from build123d import *

# Parameters (mm, degrees)
BOSS_EXTRUDE1_DEPTH = 100
BOSS_EXTRUDE2_DEPTH = 95
CUT_EXTRUDE1_DEPTH  = 5
BOSS_EXTRUDE5_DEPTH = 85
CUT_EXTRUDE4_DEPTH  = 5
BOSS_EXTRUDE6_DEPTH = 60
CUT_EXTRUDE5_DEPTH  = 40
SKETCH11_R          = 2.5
CUT_EXTRUDE6_DEPTH  = 15
SKETCH12_R          = 2.5
CUT_EXTRUDE7_DEPTH  = 15
CUT_EXTRUDE8_DEPTH  = 5
CUT_EXTRUDE9_DEPTH  = 30
CUT_EXTRUDE10_DEPTH = 5
CUT_EXTRUDE11_DEPTH = 30


with BuildPart() as part:
    # Sketch1 → Boss-Extrude1 (new body)
    with BuildSketch(Plane.XY):
        with BuildLine():
            Line((-70, 0), (-70, 30))
            Line((-70, 30), (-55, 45))
            Line((-55, 45), (-55, 55))
            Line((-55, 55), (-70, 70))
            Line((-70, 70), (-70, 100))
            ThreePointArc((-70, 100), (-35, 65), (0, 100))
            Line((0, 100), (0, 70))
            Line((0, 70), (-15, 55))
            Line((-15, 55), (-15, 45))
            Line((-15, 45), (0, 30))
            Line((0, 30), (0, 0))
            ThreePointArc((0, 0), (-35, 35), (-70, 0))
        make_face()
    extrude(amount=BOSS_EXTRUDE1_DEPTH)

    # Sketch2 → Boss-Extrude2 (add)
    with BuildSketch(Plane(origin=(0, 0, 0), x_dir=(-1, 0, 0), z_dir=(0, 0, -1))):
        with BuildLine():
            Line((0, 100), (10, 100))
            ThreePointArc((10, 100), (35, 75), (60, 100))
            Line((60, 100), (70, 100))
            ThreePointArc((70, 100), (35, 65), (0, 100))
        make_face()
        with BuildLine():
            Line((0, 0), (10, 0))
            ThreePointArc((10, 0), (35, 25), (60, 0))
            Line((60, 0), (70, 0))
            ThreePointArc((70, 0), (35, 35), (0, 0))
        make_face()
    extrude(amount=-BOSS_EXTRUDE2_DEPTH)

    # Sketch3 → Cut-Extrude1 (cut)
    with BuildSketch(Plane(origin=(0, 0, 0), x_dir=(-1, 0, 0), z_dir=(0, 0, -1))):
        with BuildLine():
            Line((0, 100), (10, 100))
            ThreePointArc((10, 100), (35, 75), (60, 100))
            Line((60, 100), (70, 100))
            ThreePointArc((70, 100), (35, 65), (0, 100))
        make_face()
        with BuildLine():
            Line((60, 0), (70, 0))
            ThreePointArc((70, 0), (35, 35), (0, 0))
            Line((0, 0), (10, 0))
            ThreePointArc((10, 0), (35, 25), (60, 0))
        make_face()
    extrude(amount=-CUT_EXTRUDE1_DEPTH, mode=Mode.SUBTRACT)

    # Sketch4 → Boss-Extrude5 (add)
    with BuildSketch(Plane(origin=(0, 0, 5), x_dir=(-1, 0, 0), z_dir=(0, 0, -1))):
        with BuildLine():
            Line((10, 100), (17.5, 100))
            ThreePointArc((17.5, 100), (35, 82.5), (52.5, 100))
            Line((52.5, 100), (60, 100))
            ThreePointArc((60, 100), (35, 75), (10, 100))
        make_face()
        with BuildLine():
            Line((10, 0), (17.5, 0))
            ThreePointArc((17.5, 0), (35, 17.5), (52.5, 0))
            Line((52.5, 0), (60, 0))
            ThreePointArc((60, 0), (35, 25), (10, 0))
        make_face()
    extrude(amount=-BOSS_EXTRUDE5_DEPTH)

    # Sketch7 → Cut-Extrude4 (cut)
    with BuildSketch(Plane(origin=(0, 0, 5), x_dir=(-1, 0, 0), z_dir=(0, 0, -1))):
        with BuildLine():
            ThreePointArc((52.5, 100), (35, 82.5), (17.5, 100))
            Line((17.5, 100), (10, 100))
            ThreePointArc((10, 100), (35, 75), (60, 100))
            Line((60, 100), (52.5, 100))
        make_face()
        with BuildLine():
            Line((10, 0), (17.5, 0))
            ThreePointArc((17.5, 0), (35, 17.5), (52.5, 0))
            Line((52.5, 0), (60, 0))
            ThreePointArc((60, 0), (35, 25), (10, 0))
        make_face()
    extrude(amount=-CUT_EXTRUDE4_DEPTH, mode=Mode.SUBTRACT)

    # Sketch9 → Boss-Extrude6 (add)
    with BuildSketch(Plane(origin=(0, 0, 0), x_dir=(-1, 0, 0), z_dir=(0, 0, -1))):
        Polygon((10, 40), (15, 45), (15, 55), (10, 60), align=None)
        Polygon((60, 60), (55, 55), (55, 45), (60, 40), align=None)
    extrude(amount=-BOSS_EXTRUDE6_DEPTH)

    # Sketch10 → Cut-Extrude5 (cut)
    with BuildSketch(Plane(origin=(0, 0, 0), x_dir=(-1, 0, 0), z_dir=(0, 0, -1))):
        Polygon((10, 40), (15, 45), (15, 55), (10, 60), align=None)
        Polygon((60, 40), (55, 45), (55, 55), (60, 60), align=None)
    extrude(amount=-CUT_EXTRUDE5_DEPTH, mode=Mode.SUBTRACT)

    # Sketch11 → Cut-Extrude6 (cut)
    with BuildSketch(Plane(origin=(-10, 0, 0), x_dir=(0, 0, -1), z_dir=(1, 0, 0))):
        with Locations((-50, 50)):
            Circle(SKETCH11_R)
    extrude(amount=-CUT_EXTRUDE6_DEPTH, mode=Mode.SUBTRACT)

    # Sketch12 → Cut-Extrude7 (cut)
    with BuildSketch(Plane.ZY.offset(60)):
        with Locations((50, 50)):
            Circle(SKETCH12_R)
    extrude(amount=-CUT_EXTRUDE7_DEPTH, mode=Mode.SUBTRACT)

    # Sketch13 → Cut-Extrude8 (cut)
    with BuildSketch(Plane(origin=(0, 0, 0), x_dir=(-1, 0, 0), z_dir=(0, 0, -1))):
        with BuildLine():
            Line((30, 60), (40, 60))
            ThreePointArc((40, 60), (50, 50), (40, 40))
            Line((40, 40), (30, 40))
            ThreePointArc((30, 40), (20, 50), (30, 60))
        make_face()
    extrude(amount=-CUT_EXTRUDE8_DEPTH, mode=Mode.SUBTRACT)

    # Sketch14 → Cut-Extrude9 (cut)
    with BuildSketch(Plane(origin=(0, 0, 5), x_dir=(-1, 0, 0), z_dir=(0, 0, -1))):
        with BuildLine():
            Line((30, 55), (40, 55))
            ThreePointArc((40, 55), (45, 50), (40, 45))
            Line((40, 45), (30, 45))
            ThreePointArc((30, 45), (25, 50), (30, 55))
        make_face()
    extrude(amount=-CUT_EXTRUDE9_DEPTH, mode=Mode.SUBTRACT)

    # Sketch15 → Cut-Extrude10 (cut)
    with BuildSketch(Plane.XY.offset(100)):
        with BuildLine():
            Line((-40, 60), (-30, 60))
            ThreePointArc((-30, 60), (-20, 50), (-30, 40))
            Line((-30, 40), (-40, 40))
            ThreePointArc((-40, 40), (-50, 50), (-40, 60))
        make_face()
    extrude(amount=-CUT_EXTRUDE10_DEPTH, mode=Mode.SUBTRACT)

    # Sketch16 → Cut-Extrude11 (cut)
    with BuildSketch(Plane.XY.offset(95)):
        with BuildLine():
            Line((-40, 55), (-30, 55))
            ThreePointArc((-30, 55), (-25, 50), (-30, 45))
            Line((-30, 45), (-40, 45))
            ThreePointArc((-40, 45), (-45, 50), (-40, 55))
        make_face()
    extrude(amount=-CUT_EXTRUDE11_DEPTH, mode=Mode.SUBTRACT)


solid = part.part
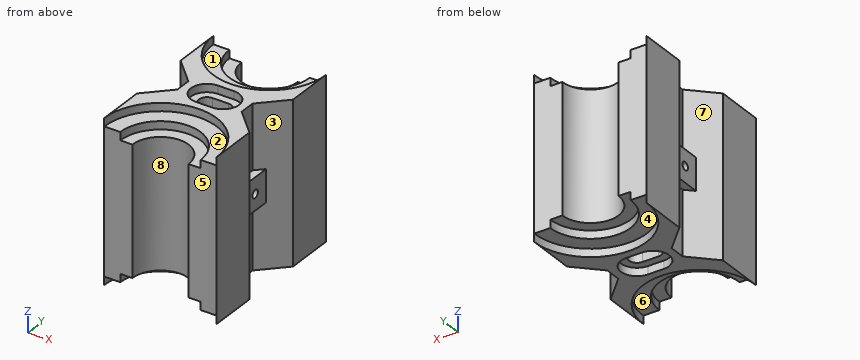
Check sheet for the modelled part. Datum: model origin and axes. Units: mm. Face numbers are marked on the shaded views. A direction names the side the tool comes from. Round coordinates to 2 decimals unless told otherwise and drop trailing zeros. Write each loop counter-clockwise with the first axis right and the second up, starting at its lowest first coordinate (ties: lowest second). Pieces come first, ordered by that corner, then holes. Notation, with made-up numbers: (69, 80.5) - (73, 80.5) arc R12 cw to (73, 97.5) - close; hole circle Ø9 at (86.5, 28.5). An arc over 180 degrees is marked (long way). Return JSON: item names as keys, results as strings.
Q1. Access from +Z, -Z, +X, -X, +Y, -Y to the whole of each face (thin tool, end or side, straight path). Record for the marked faces 1, 2, 3 and 4.
Returned:
{"face 1": "+Z, +Y", "face 2": "+Z, -Y", "face 3": "+X", "face 4": "-Z, +Y"}
Q2. Cross-section at B-B (x = -64.5). Record the boundary of the cut face in (y, z).
Returned:
{"outline": "(0, 5) - (18.83, 5) - (18.83, 0) - (35.5, 0) - (35.5, 100) - (18.83, 100) - (18.83, 95) - (0, 95) - close; (64.5, 0) - (81.17, 0) - (81.17, 5) - (100, 5) - (100, 95) - (81.17, 95) - (81.17, 100) - (64.5, 100) - close"}
Q3. Draft check along X on the marked faces 5, 6, 7 and 8. Enter one of: released by +X, released by -X, zero draft, split by the parting line, or undercut.
Returned:
{"face 5": "zero draft", "face 6": "undercut", "face 7": "released by -X", "face 8": "undercut"}
Q4. Scan lines: L1, parallel to Y at x = -53.5, z = 50; L2, parallel to Y at x = -34, z = 66; L3, parallel to Z at x = -45.5, y = 54. Record each from-to range of solid material in increasing order. Write a range as from..to.
Returned:
{"L1": "y = 0..47.5, 52.5..100", "L2": "y = 17.47..45, 55..82.53", "L3": "z = 5..95"}
Q5. Depth check by flat-ended pin: P1, Ø5.5, axis at x = -34.5, z = 1.5, coming from the +Y side; P2, Ø1.5, axis at x = -35.5, z = 98, coming from the +Y side; P3, Ø1, axis at x = -25.5, z = 58.5, coming from the -Y side. Enter the tip coordinate at first touch or a pass-through.
Returned:
{"P1": "stops at y = 65.15", "P2": "stops at y = 65.02", "P3": "stops at y = 14.36"}
Q6. Cross-section at A-A (z = 84.5). Record the boundary of the cut face in (x, y), then the cut area to 3 significant figures.
Returned:
{"outline": "(-70, 0) - (-52.5, 0) arc R17.5 cw to (-17.5, 0) - (0, 0) - (0, 30) - (-15, 45) - (-15, 55) - (0, 70) - (0, 100) - (-17.5, 100) arc R17.5 cw to (-52.5, 100) - (-70, 100) - (-70, 70) - (-55, 55) - (-55, 45) - (-70, 30) - close; hole (-40, 45) - (-30, 45) arc R5 ccw to (-30, 55) - (-40, 55) arc R5 ccw to start", "area": "5,110 mm²"}
Q7. Cross-section at C-C (z = 50). Record the boundary of the cut face in (x, y).
Returned:
{"outline": "(-70, 0) - (-52.5, 0) arc R17.5 cw to (-17.5, 0) - (0, 0) - (0, 30) - (-10, 40) - (-10, 47.5) - (-25, 47.5) - (-25, 52.5) - (-10, 52.5) - (-10, 60) - (0, 70) - (0, 100) - (-17.5, 100) arc R17.5 cw to (-52.5, 100) - (-70, 100) - (-70, 70) - (-60, 60) - (-60, 52.5) - (-45, 52.5) - (-45, 47.5) - (-60, 47.5) - (-60, 40) - (-70, 30) - close"}
Q8. Cross-section at D-D (y = 33). Record the boundary of the cut face in (x, z).
Returned:
{"outline": "(-67, 0) - (-46.66, 0) - (-46.66, 5) - (-23.34, 5) - (-23.34, 0) - (-3, 0) - (-3, 100) - (-23.34, 100) - (-23.34, 95) - (-46.66, 95) - (-46.66, 100) - (-67, 100) - close"}
